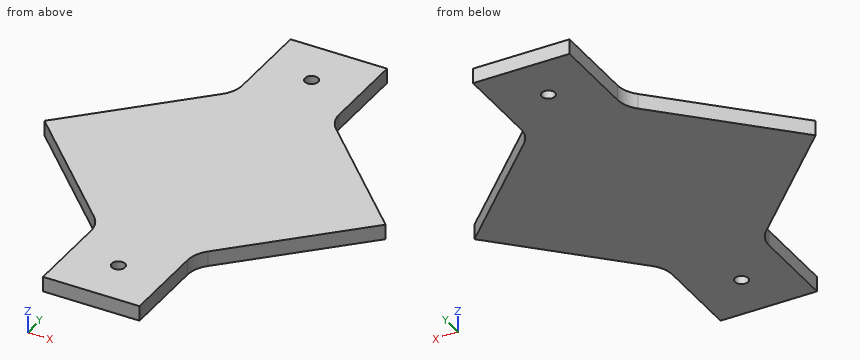
from build123d import *

# Parameters (mm, degrees)
SKETCH1_R      = 2.778125
EXTRUDE1_DEPTH = 6.35


with BuildPart() as part:
    # Sketch1 → Extrude1 (new body)
    with BuildSketch(Plane.XY):
        with BuildLine():
            Line((71.842048969, 0), (24.039743879, 47.80230509))
            ThreePointArc((24.039743879, 47.80230509), (21.286729937, 51.92248162), (20.32, 56.782561211))
            Line((20.32, 56.782561211), (20.32, 92.56248162))
            Line((20.32, 92.56248162), (-20.32, 92.56248162))
            Line((-20.32, 92.56248162), (-20.32, 56.782561211))
            ThreePointArc((-20.32, 56.782561211), (-21.286729937, 51.92248162), (-24.039743879, 47.80230509))
            Line((-24.039743879, 47.80230509), (-71.842048969, 0))
            Line((-71.842048969, 0), (-24.039743879, -47.80230509))
            ThreePointArc((-24.039743879, -47.80230509), (-21.286729937, -51.92248162), (-20.32, -56.782561211))
            Line((-20.32, -56.782561211), (-20.32, -92.56248162))
            Line((-20.32, -92.56248162), (20.32, -92.56248162))
            Line((20.32, -92.56248162), (20.32, -56.782561211))
            ThreePointArc((20.32, -56.782561211), (21.286729937, -51.92248162), (24.039743879, -47.80230509))
            Line((24.039743879, -47.80230509), (71.842048969, 0))
        make_face()
        with Locations((0, 72.24248162)):
            Circle(SKETCH1_R, mode=Mode.SUBTRACT)
        with Locations((0, -72.24248162)):
            Circle(SKETCH1_R, mode=Mode.SUBTRACT)
    extrude(amount=EXTRUDE1_DEPTH)


solid = part.part
Geometry: final body of the model. Coordinates: model frame, mm. Coordinates: 2 decimals unless noted, no trailing zeros. Write each loop counter-clockwise with the first axis right and the second up, starting at its lowest first coordinate (ties: lowest second). Pieces come first, ordered by that corner, then holes. Notation, with made-up numbers: (-0.5, 24) - (29.5, 24) arc R27 ccw to (29.5, 41) - close; hole circle Ø3 at (-3, -35). An arc over 180 degrees is marked (long way). Return JSON: item names as keys, results as strings.
Item 1: Line query: L1, parallel to Y at x = 0, z = 4.75; L2, parallel to X at y = 57, z = 3.75; L3, parallel to X at y = -73, z = 5.5. Output: solid intervals per line, ascending.
Completed:
{"L1": "y = -92.56 to -75.02, -69.46 to 69.46, 75.02 to 92.56", "L2": "x = -20.32 to 20.32", "L3": "x = -20.32 to -2.67, 2.67 to 20.32"}
Item 2: Pin query (flat end, axial travel): pin 1 Ø1.5 at (y, z) = (44, 1) entering from +X; pin 2 Ø3 at (y, z) = (7.5, 3.5) entering from -X; pin 3 Ø1.9 at (y, z) = (72, 4) entering from -X. Return the tip coordinate at first contact, or that it passes through.
Completed:
{"pin 1": "stops at x = 28.59", "pin 2": "stops at x = -65.84", "pin 3": "stops at x = -20.32"}
Item 3: Section query C-C (z = 1.75). Output: boundary loops of the cut face in (x, y), and give its area (3 significant figures).
Completed:
{"outline": "(-71.84, 0) - (-24.04, -47.8) arc R12.7 cw to (-20.32, -56.78) - (-20.32, -92.56) - (20.32, -92.56) - (20.32, -56.78) arc R12.7 cw to (24.04, -47.8) - (71.84, 0) - (24.04, 47.8) arc R12.7 cw to (20.32, 56.78) - (20.32, 92.56) - (-20.32, 92.56) - (-20.32, 56.78) arc R12.7 cw to (-24.04, 47.8) - close; hole circle Ø5.56 at (0, -72.24); hole circle Ø5.56 at (0, 72.24)", "area": "12,800 mm2"}
Item 4: Section query D-D (x = 34). Output: boundary loops of the cut face in (y, z).
Completed:
{"outline": "(-37.84, 0) - (37.84, 0) - (37.84, 6.35) - (-37.84, 6.35) - close"}
Item 5: Section query B-B (y = -78). Output: boundary loops of the cut face in (x, z).
Completed:
{"outline": "(-20.32, 0) - (20.32, 0) - (20.32, 6.35) - (-20.32, 6.35) - close"}
Item 6: Section query A-A (x = 0). Output: boundary loops of the cut face in (y, z).
Completed:
{"outline": "(-92.56, 0) - (-75.02, 0) - (-75.02, 6.35) - (-92.56, 6.35) - close; (-69.46, 0) - (69.46, 0) - (69.46, 6.35) - (-69.46, 6.35) - close; (75.02, 0) - (92.56, 0) - (92.56, 6.35) - (75.02, 6.35) - close"}
